Check sheet for the modelled part. Datum: model origin and axes. Units: mm. Round coordinates to 2 decimals unless told otherwise and drop trailing zeros. Loops run counter-clockwise (first coordinate to the right, second up) from the corner with the lowest first, then second, coordinate; pieces in that order, holes last. Notation, with made-up numbers: (-5.75, -17) -> (3.25, -17) arc R12 cw to (3.25, -13) -> close; hole circle Ø3 at (76, -37.5). An arc over 180 degrees is marked (long way). Return JSON: item names as keys, results as strings.
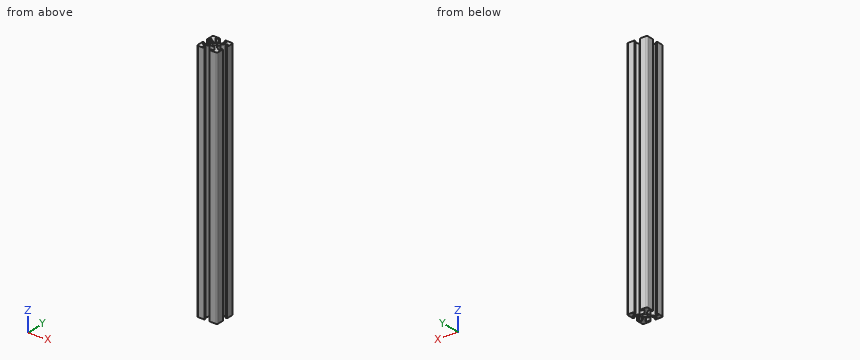
from build123d import *

# Parameters (mm, degrees)
SKETCH1_W           = 25.4
SKETCH1_H           = 25.4
BOSS_EXTRUDE1_DEPTH = 304.8
FILLET1_R           = 1.5875
HOLE1_OUTLINE_R     = 2.5527
HOLE1_DEPTH         = 304.8
SKETCH7_W           = 6.5278
SKETCH7_H           = 2.2352
CUT_EXTRUDE2_DEPTH  = 304.8
FILLET4_R           = 0.396875
CIRPATTERN2_DEPTH   = 304.8


# Read off the part's stored shape, not the designer's step: Hole1, CirPattern2
with BuildPart() as part:
    # Sketch1 → Boss-Extrude1 (new body)
    with BuildSketch(Plane.XY):
        Rectangle(SKETCH1_W, SKETCH1_H)
    extrude(amount=BOSS_EXTRUDE1_DEPTH)

    # Fillet1
    fillet1_edges = [part.edges().sort_by_distance(p)[0] for p in [
        (12.7, -12.7, 152.4),
        (-12.7, -12.7, 152.4),
        (-12.7, 12.7, 152.4),
        (12.7, 12.7, 152.4),
    ]]
    fillet(fillet1_edges, radius=FILLET1_R)

    # Hole1 outline → Hole1 (cut)
    with BuildSketch(Plane.XY):
        with Locations((0, -0.048792482)):
            Circle(HOLE1_OUTLINE_R)
    extrude(amount=HOLE1_DEPTH, mode=Mode.SUBTRACT)

    # Sketch7 → Cut-Extrude2 (cut)
    with BuildSketch(Plane.XY.offset(304.8)):
        with Locations((0, 11.5824)):
            Rectangle(SKETCH7_W, SKETCH7_H)
        Polygon((-3.175, 4.5212), (-7.3025, 10.4648), (7.3025, 10.4648), (3.175, 4.5212), align=None)
    extrude(amount=-CUT_EXTRUDE2_DEPTH, mode=Mode.SUBTRACT)

    # Fillet4
    fillet4_edges = [part.edges().sort_by_distance(p)[0] for p in [
        (-3.2639, 10.4648, 152.4),
        (-3.2639, 12.7, 152.4),
        (3.2639, 12.7, 152.4),
        (3.2639, 10.4648, 152.4),
    ]]
    fillet(fillet4_edges, radius=FILLET4_R)

    # CirPattern2 outline → CirPattern2 (cut)
    with BuildSketch(Plane.XY):
        with BuildLine():
            ThreePointArc((-3.660775, -10.562384964), (-3.380141996, -10.67862696), (-3.2639, -10.959259964))
            Line((-3.2639, -10.959259964), (-3.2639, -12.7))
            Line((-3.2639, -12.7), (3.2639, -12.7))
            Line((3.2639, -12.7), (3.2639, -10.959259964))
            ThreePointArc((3.2639, -10.959259964), (3.380141996, -10.67862696), (3.660775, -10.562384964))
            Line((3.660775, -10.562384964), (7.3025, -10.562384964))
            Line((7.3025, -10.562384964), (3.175, -4.618784964))
            Line((3.175, -4.618784964), (-3.175, -4.618784964))
            Line((-3.175, -4.618784964), (-7.3025, -10.562384964))
            Line((-7.3025, -10.562384964), (-3.660775, -10.562384964))
        make_face()
        with BuildLine():
            Line((-12.7, -3.312692482), (-10.910467482, -3.312692482))
            ThreePointArc((-10.910467482, -3.312692482), (-10.629834478, -3.428934478), (-10.513592482, -3.709567482))
            Line((-10.513592482, -3.709567482), (-10.513592482, -7.351292482))
            Line((-10.513592482, -7.351292482), (-4.569992482, -3.223792482))
            Line((-4.569992482, -3.223792482), (-4.569992482, 3.126207518))
            Line((-4.569992482, 3.126207518), (-10.513592482, 7.253707518))
            Line((-10.513592482, 7.253707518), (-10.513592482, 3.611982518))
            ThreePointArc((-10.513592482, 3.611982518), (-10.629834478, 3.331349514), (-10.910467482, 3.215107518))
            Line((-10.910467482, 3.215107518), (-12.7, 3.215107518))
            Line((-12.7, 3.215107518), (-12.7, -3.312692482))
        make_face()
        with BuildLine():
            ThreePointArc((10.513592482, -3.709567482), (10.629834478, -3.428934478), (10.910467482, -3.312692482))
            Line((10.910467482, -3.312692482), (12.7, -3.312692482))
            Line((12.7, -3.312692482), (12.7, 3.215107518))
            Line((12.7, 3.215107518), (10.910467482, 3.215107518))
            ThreePointArc((10.910467482, 3.215107518), (10.629834478, 3.331349514), (10.513592482, 3.611982518))
            Line((10.513592482, 3.611982518), (10.513592482, 7.253707518))
            Line((10.513592482, 7.253707518), (4.569992482, 3.126207518))
            Line((4.569992482, 3.126207518), (4.569992482, -3.223792482))
            Line((4.569992482, -3.223792482), (10.513592482, -7.351292482))
            Line((10.513592482, -7.351292482), (10.513592482, -3.709567482))
        make_face()
    extrude(amount=CIRPATTERN2_DEPTH, mode=Mode.SUBTRACT)


solid = part.part
Q1. Go/stop test with flat-tipped pins: pin 1 (0.5 mm diameter, centred on x = -11.5, z = 177.5, fed in from +Y); pin 2 (1.9 mm diameter, centred on y = 1.5, z = 157, fed in from +X); pin 3 (5 mm diameter, centred on y = -0.5, z = 219.5, fed in from -X). Record where each tip stops, or that it passes through.
Results list:
{"pin 1": "y = 12.69", "pin 2": "x = 4.57", "pin 3": "x = -4.57"}
Q2. Section check A-A (x = 0). Record the boundary of the cut face in (y, z).
Results list:
{"outline": "(-4.62, 0) -> (-2.6, 0) -> (-2.6, 304.8) -> (-4.62, 304.8) -> close; (2.5, 0) -> (4.52, 0) -> (4.52, 304.8) -> (2.5, 304.8) -> close"}
Q3. Material ranges on line 1 (X direction, y = -0.5, z = 290); line 2 (Y direction, x = 5.25, z = 266); line 3 (Y direction, x = 0, z = 206), recorded low to high.
Results list:
{"line 1": "-4.57 to -2.51, 2.51 to 4.57", "line 2": "-12.7 to -10.56, -7.61 to -3.7, 3.6 to 7.51, 10.46 to 12.7", "line 3": "-4.62 to -2.6, 2.5 to 4.52"}
